For this review, take the finished solid that the model builds, in its own axes (mm). A direction names the side the tool comes from. Coordinates: 2 decimals unless noted, no trailing zeros. Loops run counter-clockwise (first coordinate to the right, second up) from the corner with the lowest first, then second, coordinate; pieces in that order, holes last. Notation, with made-up numbers: (-1.5, 42) - (56.5, 42) arc R20 cw to (56.5, 70) - close; hole circle Ø10 at (-27, 38). An arc over 180 degrees is marked (long way). One line per item, written item: value. Start each with the question number.
1. For faces 1 (the face through (-20, 12, -7)), 2 (the face through (-10, 13, -7)), 3 (the face through (-19, 10, -1)), list the 3-axis set-ups (+Z, -Z, +X, -X, +Y, -Y) from which the entire face can be reached by the end or side of a thin tool; tool diameter is ignored.
2. Take a section at A-A, the plane z = -8. State the section outline as (x, y) points, and give its area (3 significant figures).
3. The part is to be moulded in two halves that separate along Z. For faces 4 (the face through (-15, 0, -5)), 5 (the face through (-15, 7, -10)), 6 (the face through (-15, 8.8, -6)), 7 (the face through (-25.88, 2.54, -6.15)), say which applies: released by +Z, released by -Z, zero draft, split by the parting line, or undercut.
4. Take a section at D-D, the plane z = -4.5. State the section outline as (x, y) points, and give its area (3 significant figures).
5. To check wall thickness, follow line 1 (X direction, y = 3.15, z = -5); line 2 (X direction, y = 17, z = -5.5); line 3 (X direction, y = 9.75, z = -2.5). State the ranges of each line that lie inside material, in increasing order. Write a range as from..to.
6. Take a section at C-C, the plane x = -25. State the section outline as (y, z) points.
7. Insertion check: pin 1 (3.5 mm diameter, centred on x = -18, z = -2, fed in from +Y); pin 2 (4 mm diameter, centred on y = 18, z = -6.5, fed in from +X); pin 3 (1.1 mm diameter, centred on y = 9.5, z = -2, fed in from -X); pin 4 (2.5 mm diameter, centred on x = -25, z = -5, fed in from -Y). Each pin has a flat end and moves straight along its axis. Give the tip position at first contact, or say it passes through.
8. Take a section at B-B, the plane y = 19.25. State the section outline as (x, z) points.
```python
from build123d import *

# Parameters (mm, degrees)
EXTRUDE_1_DEPTH     = 4
SKETCH_2_W          = 10
SKETCH_2_H          = 15
EXTRUDE_2_DEPTH     = 20
SKETCH_3_R          = 1.45
CUT_EXTRUDE_1_DEPTH = 20
SKETCH_4_W          = 6
SKETCH_4_H          = 13.2
CUT_EXTRUDE_2_DEPTH = 9.5
SKETCH_6_R          = 0.75
CUT_EXTRUDE_4_DEPTH = 3.5
SKETCH_7_W          = 10
SKETCH_7_H          = 24
CUT_EXTRUDE_5_DEPTH = 5
SKETCH_9_W          = 3
SKETCH_9_H          = 12
CUT_EXTRUDE_6_DEPTH = 10
SKETCH_11_W         = 1.5
SKETCH_11_H         = 12
CUT_EXTRUDE_7_DEPTH = 10
CUT_EXTRUDE_8_REACH = 41.699
SKETCH_13_W         = 10
SKETCH_13_H         = 5
SKETCH_19_W         = 10
SKETCH_19_H         = 2.4
EXTRUDE_6_DEPTH     = 4.8
SKETCH_20_W         = 10
SKETCH_20_H         = 2.6
EXTRUDE_7_DEPTH     = 6
FILLET_17_R         = 0.25
SKETCH_21_W         = 4
SKETCH_21_H         = 1
CUT_EXTRUDE_9_DEPTH = 5.2
EXTRUDE_8_DEPTH     = 0.4
EXTRUDE_START       = 1
SKETCH_29_W         = 10
SKETCH_29_H         = 10
SKETCH_29_R         = 1.45
EXTRUDE_9_DEPTH     = 1


with BuildPart() as part:
    # 草图1 → 凸台-拉伸1 (new body)
    with BuildSketch(Plane(origin=(0, 0, 0), x_dir=(1, 0, 0), z_dir=(0, 1, 0))):
        Polygon((-20, 0), (-20, -5), (-10, -5), (-10, 0), (0, 0), (0, 10), (-30, 10), (-30, 0), align=None)
    extrude(amount=EXTRUDE_1_DEPTH)

    # 草图2 → 凸台-拉伸2 (add)
    with BuildSketch(Plane(origin=(0, 4, 0), x_dir=(1, 0, 0), z_dir=(0, 1, 0))):
        with Locations((-15, 2.5)):
            Rectangle(SKETCH_2_W, SKETCH_2_H)
    extrude(amount=EXTRUDE_2_DEPTH)

    # 草图3 → 切除-拉伸1 (cut)
    with BuildSketch(Plane(origin=(0, 4, 0), x_dir=(1, 0, 0), z_dir=(0, 1, 0))):
        with Locations(Location((-25, 5, 0), (0, 0, 270))):
            Circle(SKETCH_3_R)
        with Locations(Location((-5, 5, 0), (0, 0, 270))):
            Circle(SKETCH_3_R)
    extrude(amount=-CUT_EXTRUDE_1_DEPTH, mode=Mode.SUBTRACT)

    # 草图4 → 切除-拉伸2 (cut)
    with BuildSketch(Plane(origin=(0, 0, -10), x_dir=(-1, 0, 0), z_dir=(0, 0, -1))):
        with Locations((15, 15.4)):
            Rectangle(SKETCH_4_W, SKETCH_4_H)
    extrude(amount=-CUT_EXTRUDE_2_DEPTH, mode=Mode.SUBTRACT)

    # 草图6 → 切除-拉伸4 (cut)
    with BuildSketch(Plane(origin=(0, 0, -0.5), x_dir=(-1, 0, 0), z_dir=(0, 0, -1))):
        with Locations((15, 20.68)):
            Circle(SKETCH_6_R)
        with Locations((15, 10.52)):
            Circle(SKETCH_6_R)
        with Locations((15, 15.6)):
            Circle(SKETCH_6_R)
    extrude(amount=-CUT_EXTRUDE_4_DEPTH, mode=Mode.SUBTRACT)

    # 草图7 → 切除-拉伸5 (cut)
    with BuildSketch(Plane.XY.offset(5)):
        with Locations((-15, 12)):
            Rectangle(SKETCH_7_W, SKETCH_7_H)
    extrude(amount=-CUT_EXTRUDE_5_DEPTH, mode=Mode.SUBTRACT)

    # 草图9 → 切除-拉伸6 (cut)
    with BuildSketch(Plane(origin=(0, 0, -0.5), x_dir=(-1, 0, 0), z_dir=(0, 0, -1))):
        with Locations((15, 15.6)):
            Rectangle(SKETCH_9_W, SKETCH_9_H)
    extrude(amount=-CUT_EXTRUDE_6_DEPTH, mode=Mode.SUBTRACT)

    # 草图11 → 切除-拉伸7 (cut)
    with BuildSketch(Plane(origin=(0, 0, -0.5), x_dir=(-1, 0, 0), z_dir=(0, 0, -1))):
        with Locations((17.25, 15.6)):
            Rectangle(SKETCH_11_W, SKETCH_11_H)
        with Locations((12.75, 15.6)):
            Rectangle(SKETCH_11_W, SKETCH_11_H)
    extrude(amount=-CUT_EXTRUDE_7_DEPTH, mode=Mode.SUBTRACT)

    # 切除-拉伸8: up to this face of the body (flat: up to its plane)
    cut_extrude_8_end = Plane(part.part.faces().sort_by_distance((-5, 4, -9.858578644))[0])
    # 草图13 → 切除-拉伸8 (cut, up to the picked face)
    with BuildSketch(Plane(origin=(0, 24, 0), x_dir=(1, 0, 0), z_dir=(0, 1, 0)), mode=Mode.PRIVATE) as cut_extrude_8_sk1:
        with Locations((-15, 2.5)):
            Rectangle(SKETCH_13_W, SKETCH_13_H)
    cut_extrude_8_tool1 = split(extrude(cut_extrude_8_sk1.sketch, amount=-CUT_EXTRUDE_8_REACH, mode=Mode.PRIVATE), bisect_by=cut_extrude_8_end, keep=Keep.BOTH, mode=Mode.PRIVATE)
    add(cut_extrude_8_tool1.solids().sort_by(Axis((-15, 24, -2.5), (0, -1, 0)))[0], mode=Mode.SUBTRACT)

    # 草图19 → 凸台-拉伸6 (add)
    with BuildSketch(Plane(origin=(0, 4, 0), x_dir=(1, 0, 0), z_dir=(0, 1, 0))):
        with Locations((-15, 3.8)):
            Rectangle(SKETCH_19_W, SKETCH_19_H)
    extrude(amount=EXTRUDE_6_DEPTH)

    # 草图20 → 凸台-拉伸7 (add)
    with BuildSketch(Plane(origin=(0, 4, 0), x_dir=(1, 0, 0), z_dir=(0, 1, 0))):
        with Locations((-15, 1.3)):
            Rectangle(SKETCH_20_W, SKETCH_20_H)
    extrude(amount=EXTRUDE_7_DEPTH)

    # 圆角17
    fillet_17_edges = [part.edges().sort_by_distance(p)[0] for p in [
        (-12, 15.4, -10),
        (-15, 8.8, -10),
        (-18, 15.4, -10),
        (-15, 22, -10),
    ]]
    fillet(fillet_17_edges, radius=FILLET_17_R)

    # 草图21 → 切除-拉伸9 (cut)
    with BuildSketch(Plane.XY):
        with Locations((-15, 9.5)):
            Rectangle(SKETCH_21_W, SKETCH_21_H)
    extrude(amount=-CUT_EXTRUDE_9_DEPTH, mode=Mode.SUBTRACT)

    # 草图22 → 凸台-拉伸8 (add)
    with BuildSketch(Plane(origin=(0, 0, -2.6), x_dir=(-1, 0, 0), z_dir=(0, 0, -1))):
        Polygon((17, 9), (13, 9), (13, 10), (10, 10), (10, 8.8), (20, 8.8), (20, 10), (17, 10), align=None)
    extrude(amount=EXTRUDE_8_DEPTH)

    # 草图29 → 凸台-拉伸9 (add)
    # profile 1 of 2: a face of its own
    with BuildSketch(Plane(origin=(0, 4, 0), x_dir=(1, 0, 0), z_dir=(0, 1, 0)).offset(EXTRUDE_START)):
        with Locations((-25, 5)):
            Rectangle(SKETCH_29_W, SKETCH_29_H)
        with Locations(Location((-25, 5, 0), (0, 0, 270))):
            Circle(SKETCH_29_R, mode=Mode.SUBTRACT)
    # profile 2 of 2: a face of its own
    with BuildSketch(Plane(origin=(0, 4, 0), x_dir=(1, 0, 0), z_dir=(0, 1, 0)).offset(EXTRUDE_START)):
        with Locations((-5, 5)):
            Rectangle(SKETCH_29_W, SKETCH_29_H)
        with Locations(Location((-5, 5, 0), (0, 0, 270))):
            Circle(SKETCH_29_R, mode=Mode.SUBTRACT)
    extrude(amount=-EXTRUDE_9_DEPTH)


solid = part.part
```
Solutions:
1. face 1: +Z, -Z, -X, +Y
1. face 2: +Z, -Z, +X, +Y
1. face 3: +Z, +X, -X, +Y
2. outline: (-30, 0) - (0, 0) - (0, 5) - (-10, 5) - (-10, 24) - (-20, 24) - (-20, 5) - (-30, 5) - close; hole (-18, 8.8) - (-12, 8.8) - (-12, 22) - (-18, 22) - close
2. area: 261 mm2
3. face 4: zero draft
3. face 5: released by -Z
3. face 6: undercut
3. face 7: undercut
4. outline: (-30, 0) - (-26.36, 0) - (-26.36, 5) - (-30, 5) - close; (-23.64, 0) - (-6.36, 0) - (-6.36, 5) - (-10, 5) - (-10, 8.8) - (-20, 8.8) - (-20, 5) - (-23.64, 5) - close; (-3.64, 0) - (0, 0) - (0, 5) - (-3.64, 5) - close
4. area: 161 mm2
5. line 1: -30..-26.45, -23.55..-6.45, -3.55..0
5. line 2: -20..-18, -12..-10
5. line 3: -20..-17, -13..-10
6. outline: (0, -10) - (5, -10) - (5, -6.45) - (0, -6.45) - close; (0, -3.55) - (5, -3.55) - (5, 0) - (0, 0) - close
7. pin 1: y = 10
7. pin 2: x = -10
7. pin 3: x = -20
7. pin 4: through
8. outline: (-20, -10) - (-18.25, -10) arc R0.25 ccw to (-18, -9.75) - (-18, -5) - (-20, -5) - close; (-12, -9.75) arc R0.25 ccw to (-11.75, -10) - (-10, -10) - (-10, -5) - (-12, -5) - close
